```python
from build123d import *

# Parameters (mm, degrees)
F0_R     = 10.9
F1_DEPTH = 5


with BuildPart() as f1:
    # F0 (on Right) → F1 (new body)
    with BuildSketch(Plane.YZ):
        with BuildLine():
            Line((-9.16856, 27.604424), (-8.306591, 17.065519))
            ThreePointArc((-8.306591, 17.065519), (-8.74893, 15.639796), (-10.055313, 14.917501))
            ThreePointArc((-10.055313, 14.917501), (-17.028002, 10.161932), (-17.199707, 1.723666))
            ThreePointArc((-17.199707, 1.723666), (-17.107939, 0.1831), (-18.140222, -0.964137))
            Line((-18.140222, -0.964137), (-28.490412, -5.862006))
            ThreePointArc((-28.490412, -5.862006), (-32.119144, -6.115317), (-34.95924, -3.842497))
            Line((-34.95924, -3.842497), (-35.498432, -2.908589))
            ThreePointArc((-35.498432, -2.908589), (-37.504185, -1.467645), (-39.911359, -2.019799))
            ThreePointArc((-39.911359, -2.019799), (-46.943646, -13.068777), (-45.092936, -26.034418))
            ThreePointArc((-45.092936, -26.034418), (-34.789716, -34.120001), (-21.704877, -33.554351))
            ThreePointArc((-21.704877, -33.554351), (-20.02311, -31.745754), (-20.268128, -29.28825))
            Line((-20.268128, -29.28825), (-20.80732, -28.354341))
            ThreePointArc((-20.80732, -28.354341), (-21.355591, -24.758336), (-19.321852, -21.742418))
            Line((-19.321852, -21.742418), (-10.625877, -15.726479))
            ThreePointArc((-10.625877, -15.726479), (-9.169996, -15.396694), (-7.891278, -16.166907))
            ThreePointArc((-7.891278, -16.166907), (-0.286491, -19.827648), (7.107115, -15.757216))
            ThreePointArc((7.107115, -15.757216), (8.3954, -14.90746), (9.905079, -15.227825))
            Line((9.905079, -15.227825), (19.321852, -21.742418))
            ThreePointArc((19.321852, -21.742418), (21.355591, -24.758336), (20.80732, -28.354341))
            Line((20.80732, -28.354341), (20.268128, -29.28825))
            ThreePointArc((20.268128, -29.28825), (20.02311, -31.745754), (21.704877, -33.554351))
            ThreePointArc((21.704877, -33.554351), (34.789716, -34.120001), (45.092936, -26.034418))
            ThreePointArc((45.092936, -26.034418), (46.943646, -13.068777), (39.911359, -2.019799))
            ThreePointArc((39.911359, -2.019799), (37.504185, -1.467645), (35.498432, -2.908589))
            Line((35.498432, -2.908589), (34.95924, -3.842497))
            ThreePointArc((34.95924, -3.842497), (32.119144, -6.115317), (28.490412, -5.862006))
            Line((28.490412, -5.862006), (18.932469, -1.339041))
            ThreePointArc((18.932469, -1.339041), (17.918926, -0.243103), (17.946592, 1.249406))
            ThreePointArc((17.946592, 1.249406), (17.314492, 9.665716), (10.092592, 14.03355))
            ThreePointArc((10.092592, 14.03355), (8.712539, 14.724359), (8.235144, 16.191962))
            Line((8.235144, 16.191962), (9.16856, 27.604424))
            ThreePointArc((9.16856, 27.604424), (10.763552, 30.873653), (14.15192, 32.196838))
            Line((14.15192, 32.196838), (15.230304, 32.196838))
            ThreePointArc((15.230304, 32.196838), (17.481075, 33.213399), (18.206482, 35.574151))
            ThreePointArc((18.206482, 35.574151), (12.15393, 47.188779), (0, 52.068837))
            ThreePointArc((0, 52.068837), (-12.15393, 47.188779), (-18.206482, 35.574151))
            ThreePointArc((-18.206482, 35.574151), (-17.481075, 33.213399), (-15.230304, 32.196838))
            Line((-15.230304, 32.196838), (-14.15192, 32.196838))
            ThreePointArc((-14.15192, 32.196838), (-10.763552, 30.873653), (-9.16856, 27.604424))
        make_face()
        Polygon((-30.1891, -26.341452), (-37.906917, -27.199435), (-42.50886, -20.944601), (-39.392987, -13.831784), (-31.67517, -12.973801), (-27.073227, -19.228635), align=None, mode=Mode.SUBTRACT)
        Polygon((-23.427465, -18.009187), (-27.310145, -11.284187), (-23.427465, -4.559187), (-15.662104, -4.559187), (-11.779423, -11.284187), (-15.662104, -18.009187), align=None, mode=Mode.SUBTRACT)
        Polygon((37.906917, -12.973801), (42.50886, -19.228635), (39.392987, -26.341452), (31.67517, -27.199435), (27.073227, -20.944601), (30.1891, -13.831784), align=None, mode=Mode.SUBTRACT)
        Circle(F0_R, mode=Mode.SUBTRACT)
        Polygon((27.310145, -11.284187), (23.427465, -18.009187), (15.662104, -18.009187), (11.779423, -11.284187), (15.662104, -4.559187), (23.427465, -4.559187), align=None, mode=Mode.SUBTRACT)
        Polygon((-7.765361, 22.568373), (-3.882681, 29.293373), (3.882681, 29.293373), (7.765361, 22.568373), (3.882681, 15.843373), (-3.882681, 15.843373), align=None, mode=Mode.SUBTRACT)
        Polygon((-3.115874, 33.06042), (-7.717817, 39.315254), (-4.601943, 46.428071), (3.115874, 47.286054), (7.717817, 41.03122), (4.601943, 33.918403), align=None, mode=Mode.SUBTRACT)
    extrude(amount=F1_DEPTH)


solid = f1.part
```
CAD build for the part. Positions are in the model's coordinates, mm. A direction names the side the tool comes from. Round coordinates to 2 decimals unless told otherwise and drop trailing zeros. Order: outer loops, then holes, each group sorted by start corner. A loop starts at its lowest first (then second) coordinate and runs counter-clockwise, first axis right, second up. Notation, with made-up numbers: (56.5, 37) - (92.5, 37) arc R16 ccw to (92.5, 52) - close; hole circle Ø2 at (-19, 26.25). An arc over 180 degrees is marked (long way). Use CSV: the item, a comma, the result in double quotes. Start each with the question number.
1) Pin check, flat tips, straight feed: pin 1 Ø3 at (x, y) = (2.5, 6.5) entering from +Z; pin 2 Ø1.2 at (x, y) = (3.5, 14.5) entering from -Z; pin 3 Ø1.2 at (x, y) = (2, -15) entering from -Z. Stop position of each tip, or through.
2) Wall check: L1, parallel to Y at x = 3.95, z = -2 (3 decimals); L2, parallel to Z at x = 1.6, y = 0; L3, parallel to Y at x = 2.4, z = -21. Give the ranges that are in metal, low to high. Write a range as [from, to].
3) Saw through at C-C (x = 3.6). Count the separate pieces of the cut face and the enclosed holes in it, and give its area (3 significant figures).
4) Tool access for faces 4 (the cylindrical face through (2.46, -0.41, -19.83)), 5 (the flat face through (2.465, 23.778, -3.632)), 6 (the flat face through (2.46, -0.8, 46.85)): list every direction of +Z, -Z, +X, -X, +Y, -Y with a clear straight run to the whole face (end or side of a thin tool).
5) Two-plate mould, pull along Y, no slides. Class faces 1 (the flat face through (0, -7, 9)), 2 (the flat face through (2.465, -5.797, 19.159)), 3 (the cylindrical face through (2.5, -17.1, 0.2)): pulls with the +Y half, pulls with the -Y half, needs draft (parallel to the pull), parting line crosses it, or undercut.
6) Saw through at A-A (z = 37). List the corners of the cut face in (x, y).
7) Saw through at B-B (z = -24.5). List the corners of the cut face in (x, y).
Values follow:
1,pin 1,"stops at z = 51.25"
1,pin 2,"stops at z = -18.82"
1,pin 3,"stops at z = -19.17"
2,L1,"y = [-39.885, -36.308], [-20.329, -10.715], [10.715, 20.329], [36.308, 39.885]"
2,L2,"z = [-19.82, -10.9], [10.9, 15.84], [29.29, 33.41], [46.94, 52.07]"
2,L3,"y = [-46.95, -42.47], [-27.85, -18.25], [18.25, 27.11], [41.73, 46.95]"
3,separate pieces,"1"
3,enclosed holes,"7"
3,area,"2,290 mm2"
4,face 4,"-Z, +X, -X"
4,face 5,"+Z, +X, -X"
4,face 6,"+X, -X"
5,face 1,"needs draft"
5,face 2,"undercut"
5,face 3,"pulls with the -Y half"
6,outline,"(0, -17.97) - (5, -17.97) - (5, -6.01) - (0, -6.01) - close; (0, 5.95) - (5, 5.95) - (5, 17.97) - (0, 17.97) - close"
7,outline,"(0, -45.84) - (5, -45.84) - (5, -39.89) - (0, -39.89) - close; (0, -29.38) - (5, -29.38) - (5, -21.29) - (0, -21.29) - close; (0, 21.29) - (5, 21.29) - (5, 29.69) - (0, 29.69) - close; (0, 40.2) - (5, 40.2) - (5, 45.84) - (0, 45.84) - close"
